from build123d import *


with BuildPart() as part:
    # Szkic1 → Obrót1 (revolve)
    with BuildSketch(Plane.XY, mode=Mode.PRIVATE) as obr_t1_sk:
        with BuildLine():
            Line((-15.825105288, -45.893649888), (-20.325105288, -45.893649888))
            Line((-20.325105288, -45.893649888), (-20.325105288, -46.893649888))
            ThreePointArc((-20.325105288, -46.893649888), (-18.825105288, -48.393649888), (-20.325105288, -49.893649888))
            Line((-20.325105288, -49.893649888), (-20.325105288, -50.893649888))
            Line((-20.325105288, -50.893649888), (-15.825105288, -50.893649888))
            Line((-15.825105288, -50.893649888), (-15.825105288, -49.893649888))
            ThreePointArc((-15.825105288, -49.893649888), (-17.325105288, -48.393649888), (-15.825105288, -46.893649888))
            Line((-15.825105288, -46.893649888), (-15.825105288, -45.893649888))
        make_face()
    revolve(obr_t1_sk.sketch.rotate(Axis((19.531131842, -70.893649888, 0), (-1, 0, 0)), 90), axis=Axis((19.531131842, -70.893649888, 0), (-1, 0, 0)))


solid = part.part
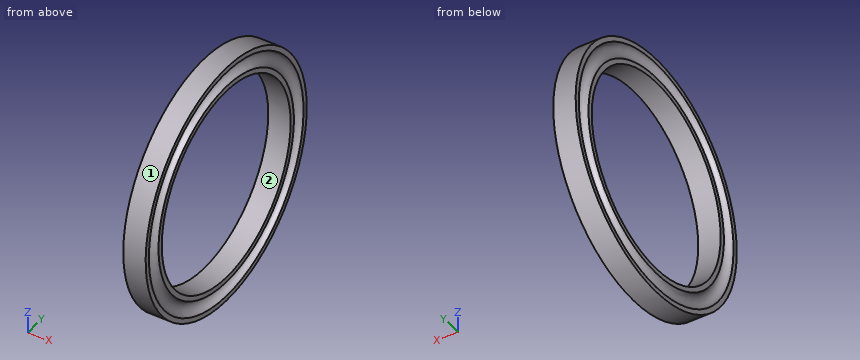
Geometry check sheet. Reference: the model listing, model coordinates, mm. Face numbers are marked on the shaded views. Give positions to 0.01 mm unless a question says otherwise; leave off trailing zeros. Write each loop counter-clockwise with the first axis right and the second up, starting at its lowest first coordinate (ties: lowest second). Pieces come first, ordered by that corner, then holes. Notation, with made-up numbers: (89, 22.25) - (146, 22.25) arc R20 ccw to (146, 42.25) - close; hole circle Ø8 at (7.5, 30.25). An arc over 180 degrees is marked (long way). Put each result on its own line as item: value.
1. Sectioned sample at C-C, the plane x = -19.55. Enter the section's corners in (y, z).
Ans:
outline: circle Ø50 at (-70.89, 0); circle Ø42.43 at (-70.89, 0); hole circle Ø47.57 at (-70.89, 0); hole circle Ø40 at (-70.89, 0)
2. Sectioned sample at B-B, the plane x = -16.65. Enter the section's corners in (y, z), plus the area to 3 significant figures.
Ans:
outline: circle Ø50 at (-70.89, 0); circle Ø42.49 at (-70.89, 0); hole circle Ø47.51 at (-70.89, 0); hole circle Ø40 at (-70.89, 0)
area: 353 mm²
3. Draft check along Z on the marked faces 1 and 2. Enter one of: +Z half, -Z half, draft (parallel to the pull), parting line (faces both ways), or undercut.
Ans:
face 1: parting line
face 2: undercut
4. Go/stop test with flat-tipped pins: pin 1 (2 mm diameter, centred on x = -19.5, y = -76, fed in from -Z); pin 2 (2 mm diameter, centred on x = -18, y = -51.5, fed in from -Z); pin 3 (1.5 mm diameter, centred on x = -19, y = -86, fed in from -Z). Record where each tip stops, or that it passes through.
Ans:
pin 1: stops at z = -24.66
pin 2: stops at z = -16.93
pin 3: stops at z = -20.47
5. Thickness scan on line 1 (Z direction, x = -17.2, y = -69.5); line 2 (Y direction, x = -16.35, z = 1); line 3 (Z direction, x = -16.1, y = -59.5). Record the ranges inside material, lowest first.
Ans:
line 1: z = -24.96 to -23.06, -21.86 to -19.95, 19.95 to 21.86, 23.06 to 24.96
line 2: y = -95.87 to -94.78, -91.96 to -90.87, -50.92 to -49.82, -47.01 to -45.91
line 3: z = -22.25 to -21.09, -17.67 to -16.44, 16.44 to 17.67, 21.09 to 22.25
6. Sectioned sample at A-A, the plane z = 0. Enter the section's corners in (x, y).
Ans:
outline: (-20.33, -95.89) - (-15.83, -95.89) - (-15.83, -94.89) arc R1.5 cw to (-15.83, -91.89) - (-15.83, -90.89) - (-20.33, -90.89) - (-20.33, -91.89) arc R1.5 cw to (-20.33, -94.89) - close; (-20.33, -50.89) - (-15.83, -50.89) - (-15.83, -49.89) arc R1.5 cw to (-15.83, -46.89) - (-15.83, -45.89) - (-20.33, -45.89) - (-20.33, -46.89) arc R1.5 cw to (-20.33, -49.89) - close
